from build123d import *

# Parameters (mm, degrees)
SKETCH1_R                = 57
BOSS_EXTRUDE1_DEPTH      = 3
SKETCH2_R                = 2
CUT_EXTRUDE1_DEPTH       = 81.665977958
CIRPATTERN1_COUNT        = 6
SKETCH5_R                = 3.25
BOSS_EXTRUDE2_DEPTH      = 5
SKETCH4_R                = 16.5
CUT_EXTRUDE3_DEPTH       = 81.765091469
SKETCH8_R                = 2
CUT_EXTRUDE4_DEPTH       = 82.006172604
SKETCH9_R                = 3
CUT_EXTRUDE5_DEPTH       = 2.5
CUT_EXTRUDE6_DEPTH       = 82.006172604
FILLET1_R                = 2
CIRPATTERN2_COUNT        = 6
FILLET1_OF_CIRPATTERN2_R = 2


with BuildPart() as part:
    # Sketch1 → Boss-Extrude1 (new body)
    with BuildSketch(Plane(origin=(0, 0, 0), x_dir=(1, 0, 0), z_dir=(0, 1, 0))):
        with Locations(Location((0, 0, 0), (0, 0, 270))):
            Circle(SKETCH1_R)
    extrude(amount=BOSS_EXTRUDE1_DEPTH)

    # Sketch2 → Cut-Extrude1 (cut, through all)
    with BuildSketch(Plane(origin=(0, 3, 0), x_dir=(1, 0, 0), z_dir=(0, 1, 0))):
        with Locations(Location((0, 46.5, 0), (0, 0, 270))):
            Circle(SKETCH2_R)
    cut_extrude1 = extrude(amount=-CUT_EXTRUDE1_DEPTH, mode=Mode.SUBTRACT)

    # CirPattern1: Cut-Extrude1 ×6 about axis
    cirpattern1_axis = Axis((0, 0, 0), (0, 1, 0))
    for i in range(1, CIRPATTERN1_COUNT):
        add(cut_extrude1.rotate(cirpattern1_axis, i * 360 / CIRPATTERN1_COUNT), mode=Mode.SUBTRACT)

    # Sketch5 → Boss-Extrude2 (add)
    with BuildSketch(Plane.XZ):
        with Locations(Location((0, 46.5, 0), (0, 0, 90))):
            Circle(SKETCH5_R)
        with Locations(Location((40.270181276, 23.25, 0), (0, 0, 90))):
            Circle(SKETCH5_R)
        with Locations(Location((40.270181276, -23.25, 0), (0, 0, 90))):
            Circle(SKETCH5_R)
        with Locations(Location((0, -46.5, 0), (0, 0, 90))):
            Circle(SKETCH5_R)
        with Locations(Location((-40.270181276, -23.25, 0), (0, 0, 90))):
            Circle(SKETCH5_R)
        with Locations(Location((-40.270181276, 23.25, 0), (0, 0, 90))):
            Circle(SKETCH5_R)
    extrude(amount=BOSS_EXTRUDE2_DEPTH)

    # Sketch4 → Cut-Extrude3 (cut, through all)
    with BuildSketch(Plane.XZ):
        with Locations(Location((0, 0, 0), (0, 0, 270))):
            Circle(SKETCH4_R)
    extrude(amount=-CUT_EXTRUDE3_DEPTH, mode=Mode.SUBTRACT)

    # Sketch8 → Cut-Extrude4 (cut, through all)
    with BuildSketch(Plane(origin=(0, 3, 0), x_dir=(1, 0, 0), z_dir=(0, 1, 0))):
        with Locations(Location((-40.270181276, -23.25, 0), (0, 0, 270))):
            Circle(SKETCH8_R)
        with Locations(Location((0, -46.5, 0), (0, 0, 270))):
            Circle(SKETCH8_R)
        with Locations(Location((40.270181276, -23.25, 0), (0, 0, 270))):
            Circle(SKETCH8_R)
        with Locations(Location((40.270181276, 23.25, 0), (0, 0, 270))):
            Circle(SKETCH8_R)
        with Locations(Location((0, 46.5, 0), (0, 0, 270))):
            Circle(SKETCH8_R)
        with Locations(Location((-40.270181276, 23.25, 0), (0, 0, 270))):
            Circle(SKETCH8_R)
    extrude(amount=-CUT_EXTRUDE4_DEPTH, mode=Mode.SUBTRACT)

    # Sketch9 → Cut-Extrude5 (cut)
    with BuildSketch(Plane(origin=(0, 3, 0), x_dir=(1, 0, 0), z_dir=(0, 1, 0))):
        with Locations(Location((-40.270181276, 23.25, 0), (0, 0, 270))):
            Circle(SKETCH9_R)
        with Locations(Location((0, 46.5, 0), (0, 0, 270))):
            Circle(SKETCH9_R)
        with Locations(Location((40.270181276, 23.25, 0), (0, 0, 270))):
            Circle(SKETCH9_R)
        with Locations(Location((40.270181276, -23.25, 0), (0, 0, 270))):
            Circle(SKETCH9_R)
        with Locations(Location((0, -46.5, 0), (0, 0, 270))):
            Circle(SKETCH9_R)
        with Locations(Location((-40.270181276, -23.25, 0), (0, 0, 270))):
            Circle(SKETCH9_R)
    extrude(amount=-CUT_EXTRUDE5_DEPTH, mode=Mode.SUBTRACT)

    # Sketch10 → Cut-Extrude6 (cut, through all)
    with BuildSketch(Plane(origin=(0, 3, 0), x_dir=(1, 0, 0), z_dir=(0, 1, 0))):
        with BuildLine():
            Line((4.849468416, 30.618338558), (7.743506019, 48.890572859))
            ThreePointArc((7.743506019, 48.890572859), (24.75, 42.868257487), (38.468725092, 31.151359357))
            Line((38.468725092, 31.151359357), (24.091524805, 19.508932123))
            ThreePointArc((24.091524805, 19.508932123), (15.5, 26.846787517), (4.849468416, 30.618338558))
        make_face()
    cut_extrude6 = extrude(amount=-CUT_EXTRUDE6_DEPTH, mode=Mode.SUBTRACT)

    # Fillet1
    fillet1_edges = [part.edges().sort_by_distance(p)[0] for p in [
        (24.091524805, 1.5, -19.508932123),
        (4.849468416, 1.5, -30.618338558),
        (7.743506019, 1.5, -48.890572859),
        (38.468725092, 1.5, -31.151359357),
    ]]
    fillet(fillet1_edges, radius=FILLET1_R)

    # CirPattern2: Cut-Extrude6 ×6 about axis
    cirpattern2_axis = Axis((0, 0, 0), (0, 1, 0))
    for i in range(1, CIRPATTERN2_COUNT):
        add(cut_extrude6.rotate(cirpattern2_axis, i * 360 / CIRPATTERN2_COUNT), mode=Mode.SUBTRACT)

    # Fillet1 of CirPattern2
    fillet1_of_cirpattern2_edges = [part.edges().sort_by_distance(p)[0] for p in [
        (-4.849468416, 1.5, -30.618338558),
        (-24.091524805, 1.5, -19.508932123),
        (-38.468725092, 1.5, -31.151359357),
        (-7.743506019, 1.5, -48.890572859),
        (-28.940993221, 1.5, -11.109406436),
        (-28.940993221, 1.5, 11.109406436),
        (-46.212231112, 1.5, 17.739213502),
        (-46.212231112, 1.5, -17.739213502),
        (-24.091524805, 1.5, 19.508932123),
        (-4.849468416, 1.5, 30.618338558),
        (-7.743506019, 1.5, 48.890572859),
        (-38.468725092, 1.5, 31.151359357),
        (4.849468416, 1.5, 30.618338558),
        (24.091524805, 1.5, 19.508932123),
        (38.468725092, 1.5, 31.151359357),
        (7.743506019, 1.5, 48.890572859),
        (28.940993221, 1.5, 11.109406436),
        (28.940993221, 1.5, -11.109406436),
        (46.212231112, 1.5, -17.739213502),
        (46.212231112, 1.5, 17.739213502),
    ]]
    fillet(fillet1_of_cirpattern2_edges, radius=FILLET1_OF_CIRPATTERN2_R)


solid = part.part
CAD build for the part. Positions are in the model's coordinates, mm. A direction names the side the tool comes from. Coordinates: 2 decimals unless noted, no trailing zeros. Loops run counter-clockwise (first coordinate to the right, second up) from the corner with the lowest first, then second, coordinate; pieces in that order, holes last. Notation, with made-up numbers: (54.25, 6.25) - (99.25, 6.25) arc R21 cw to (99.25, 30.25) - close; hole circle Ø7 at (64.5, 26). An arc over 180 degrees is marked (long way). Write item = value, one per line. Start each with the question number.
Q1. Drill centre lines: L1, parallel to X at y = -3.5, z = -23.25; L2, parallel to X at y = 1, z = -44; L3, parallel to X at y = 2.75, z = 27. Where is each one in solid material? Low to high.
Q2. Cut at B-B, the plane y = -2.5. Give the number of separate pieces and of enclosed holes in the cut face, then the cut area to 3 significant figures.
Q3. Flat gauge pins, fed straight in: pin 1 Ø1 at (x, z) = (40.5, 19) entering from -Y; pin 2 Ø1.8 at (x, z) = (-1, 48) entering from +Y; pin 3 Ø1.5 at (x, y) = (-2, 1) entering from +Z. Where does each tip first touch, or does it go through?
Q4. Cut at A-A, the plane z = 0. List the corners of the cut face in (x, y), then the cut area to 3 significant figures.
Q5. Cut at C-C, the plane x = -35. List the corners of the cut face in (y, z), then the cut area to 3 significant figures.
Q6. Pull direction X, two halves, no side cores. Call faces 4 (the cylindrical face through (-24.17, 1.48, -20.29)), 5 (the cylindrical face through (1.245, -2.465, -43.498)), 6 (the flat face through (-37.43, 1.52, 14.37)), 7 (the flat face through (-39, -5, -25)): pulls with the +X half, pulls with the -X half, needs draft (parallel to the pull), parting line crosses it, or undercut.
Q7. Which spindle directions (+Z, -Z, +X, -X, +Y, -Y) get a long thin tool onto all of the face, cutting with end or side? Do faces 1 (the flat face through (38, 0.5, -23)), 2 (the cylindrical face through (-37.614, 1.479, -31.231)), 3 (the cylindrical face through (-37.097, -2.465, 22.545)). Say none if no direction does.
Computed:
q1.L1 = -43.52 to -42.27, -38.27 to -37.02, 37.02 to 38.27, 42.27 to 43.52
q1.L2 = -36.24 to -22.68, -6.97 to -1.66, 1.66 to 6.97, 22.68 to 36.24
q1.L3 = -50.2 to -33.34, -15.23 to 15.23, 33.34 to 50.2
q2.separate_pieces = 6
q2.enclosed_holes = 6
q2.area = 124 mm²
q3.pin_1 = 0
q3.pin_2 = 0.5
q3.pin_3 = 56.99
q4.outline = (-57, 0) - (-49.5, 0) - (-49.5, 3) - (-57, 3) - close; (-31, 0) - (-16.5, 0) - (-16.5, 3) - (-31, 3) - close; (16.5, 0) - (31, 0) - (31, 3) - (16.5, 3) - close; (49.5, 0) - (57, 0) - (57, 3) - (49.5, 3) - close
q4.area = 132 mm²
q5.outline = (0, -44.99) - (3, -44.99) - (3, -35) - (0, -35) - close; (0, -28.34) - (3, -28.34) - (3, -13.44) - (0, -13.44) - close; (0, 13.44) - (3, 13.44) - (3, 28.34) - (0, 28.34) - close; (0, 35) - (3, 35) - (3, 44.99) - (0, 44.99) - close
q5.area = 149 mm²
q6.face_4 = undercut
q6.face_5 = parting line crosses it
q6.face_6 = undercut
q6.face_7 = needs draft
q7.face_1 = +Y
q7.face_2 = +Y, -Y
q7.face_3 = -Y
